Geometry: final body of the model. Coordinates: model frame, mm. A direction names the side the tool comes from. Coordinates: 2 decimals unless noted, no trailing zeros. Loops run counter-clockwise (first coordinate to the right, second up) from the corner with the lowest first, then second, coordinate; pieces in that order, holes last. Notation, with made-up numbers: M 9.25,31.5 L 68.25,31.5 A25 ccw 68.25,56.5 Z; hole C 49,84.25 d8. An arc over 180 degrees is marked long. Write each question's results on one line, items separated by ' | '. Start each with the question number.
from build123d import *

# Parameters (mm, degrees)
F1_W     = 40
F1_H     = 33
F3_DEPTH = 1275
F2_W     = 80
F2_H     = 100
F4_DEPTH = 25
F6_DEPTH = 25


with BuildPart() as f3:
    # F1 (on Right) → F3 (new body, symmetric)
    with BuildSketch(Plane.YZ):
        Polygon((20, 33), (20, 63), (17, 66), (12, 66), (12, 80), (4, 80), (4, 66), (-4, 66), (-4, 80), (-12, 80), (-12, 66), (-17, 66), (-20, 63), (-20, 33), align=None)
        with Locations((0, 16.5)):
            Rectangle(F1_W, F1_H)
        with Locations((0, -16.5)):
            Rectangle(F1_W, F1_H)
        Polygon((20, -63), (20, -33), (-20, -33), (-20, -63), (-17, -66), (-12, -66), (-12, -52), (-4, -52), (-4, -66), (4, -66), (4, -52), (12, -52), (12, -66), (17, -66), align=None)
    extrude(amount=F3_DEPTH, both=True)

    # F2 (on Front) → F4 (cut, symmetric)
    with BuildSketch(Plane.XZ):
        with Locations((-1275, 83)):
            Rectangle(F2_W, F2_H)
        with Locations((-1275, -83)):
            Rectangle(F2_W, F2_H)
        with Locations((1275, 83)):
            Rectangle(F2_W, F2_H)
        with Locations((1275, -83)):
            Rectangle(F2_W, F2_H)
    extrude(amount=F4_DEPTH, both=True, mode=Mode.SUBTRACT)

    # F5 (on Front) → F6 (cut, symmetric)
    with BuildSketch(Plane.XZ):
        Polygon((1375, 140.368329996), (-616.2874210137, 140.368329996), (1375, -46.110641775), align=None)
    extrude(amount=F6_DEPTH, both=True, mode=Mode.SUBTRACT)


solid = f3.part
Item 1: Section C-C, the plane x = 624. Return loops of the section in (y, z), plus the area to 3 significant figures.
Item 2: Contact query for flat-ended pins moving along their axis: P1, Ø1, axis at y = -4, z = 39, coming from the -X side; P2, Ø12, axis at x = -1248.5, y = 10, coming from the +Z side; P3, Ø1, axis at x = -164.5, y = -16, coming from the +Z side. Output: stop coordinate, or through.
Item 3: Set-up query: faces 1 (the flat face through (-1255, 0, -33)), 2 (the flat face through (-1235, 0, 51)), 3 (the flat face through (-1275, 0, 0)). Return all of +Z, -Z, +X, -X, +Y, -Y with unobstructed straight access to the full face (end or side cutting, diameter ignored); none if empty.
Item 4: Section A-A, the plane x = -994. Return loops of the section in (y, z).
Item 5: Ray query, L1, parallel to Y at x = -748, z = -54; L2, parallel to Y at x = -274, z = 67; L3, parallel to Z at x = -769.5, y = -5. Return the intervals inside material, ascending. Write a range as [from, to].
Item 6: Section B-B, the plane x = 325. Return loops of the section in (y, z).
Solutions:
1) outline: M -20,-63 L -17,-66 L -12,-66 L -12,-52 L -4,-52 L -4,-66 L 4,-66 L 4,-52 L 12,-52 L 12,-66 L 17,-66 L 20,-63 L 20,24.22 L -20,24.22 Z | area: 3,380 mm²
2) P1: stops at x = -1235 | P2: stops at z = 33 | P3: stops at z = 66
3) face 1: -Z, -X, +Y, -Y | face 2: +Z, -X, +Y, -Y | face 3: +Z, -Z, -X, +Y, -Y
4) outline: M -20,-63 L -17,-66 L -12,-66 L -12,-52 L -4,-52 L -4,-66 L 4,-66 L 4,-52 L 12,-52 L 12,-66 L 17,-66 L 20,-63 L 20,63 L 17,66 L 12,66 L 12,80 L 4,80 L 4,66 L -4,66 L -4,80 L -12,80 L -12,66 L -17,66 L -20,63 Z
5) L1: y = [-20, -12], [-4, 4], [12, 20] | L2: y = [-12, -4], [4, 12] | L3: z = [-52, 80]
6) outline: M -20,-63 L -17,-66 L -12,-66 L -12,-52 L -4,-52 L -4,-66 L 4,-66 L 4,-52 L 12,-52 L 12,-66 L 17,-66 L 20,-63 L 20,52.22 L -20,52.22 Z
